For this review, take the finished solid that the model builds, in its own axes (mm). Face numbers are marked on the shaded views. A direction names the side the tool comes from. Round coordinates to 2 decimals unless told otherwise and drop trailing zeros. Write each loop counter-clockwise with the first axis right and the second up, starting at its lowest first coordinate (ties: lowest second). Pieces come first, ordered by that corner, then holes. Notation, with made-up numbers: (-22, 18.5) -> (0, 18.5) arc R9 cw to (0, 27.5) -> close; hole circle Ø6 at (-15, -9.5). An arc over 180 degrees is marked (long way). Answer in a Markdown table with one row per item. Add a question column.
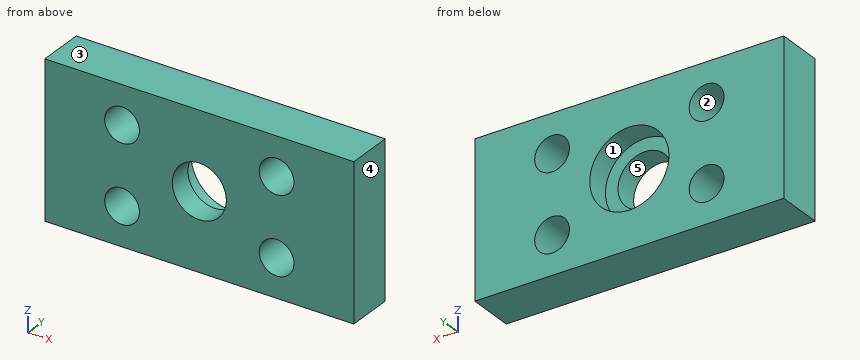
```python
from build123d import *

# Parameters (mm, degrees)
SKETCH_2_W          = 120
SKETCH_2_H          = 20
SKETCH_2_R          = 2.25
EXTRUDE_1_DEPTH     = 6
SKETCH_3_W          = 80
SKETCH_3_H          = 20
CUT_EXTRUDE_1_DEPTH = 62.12282716
SKETCH_4_R          = 5.125
CUT_EXTRUDE_2_DEPTH = 3
SKETCH_5_R          = 3.5
CUT_EXTRUDE_3_DEPTH = 61.901559914


with BuildPart() as part:
    # Эскиз2 → Бобышка-Вытянуть1 (new body)
    with BuildSketch(Plane(origin=(0, 0, 0), x_dir=(1, 0, 0), z_dir=(0, 1, 0))):
        Rectangle(SKETCH_2_W, SKETCH_2_H)
        with Locations(Location((-50, 5, 0), (0, 0, 270))):
            Circle(SKETCH_2_R, mode=Mode.SUBTRACT)
        with Locations(Location((-30, 5, 0), (0, 0, 270))):
            Circle(SKETCH_2_R, mode=Mode.SUBTRACT)
        with Locations(Location((-10, 5, 0), (0, 0, 270))):
            Circle(SKETCH_2_R, mode=Mode.SUBTRACT)
        with Locations(Location((30, 5, 0), (0, 0, 270))):
            Circle(SKETCH_2_R, mode=Mode.SUBTRACT)
        with Locations(Location((-30, -5, 0), (0, 0, 270))):
            Circle(SKETCH_2_R, mode=Mode.SUBTRACT)
        with Locations(Location((10, -5, 0), (0, 0, 270))):
            Circle(SKETCH_2_R, mode=Mode.SUBTRACT)
        with Locations(Location((50, -5, 0), (0, 0, 270))):
            Circle(SKETCH_2_R, mode=Mode.SUBTRACT)
        with Locations(Location((-50, -5, 0), (0, 0, 270))):
            Circle(SKETCH_2_R, mode=Mode.SUBTRACT)
    extrude(amount=EXTRUDE_1_DEPTH)

    # Эскиз3 → Вырез-Вытянуть1 (cut, through all)
    with BuildSketch(Plane(origin=(0, 6, 0), x_dir=(1, 0, 0), z_dir=(0, 1, 0))):
        with Locations((20, 0)):
            Rectangle(SKETCH_3_W, SKETCH_3_H)
    extrude(amount=-CUT_EXTRUDE_1_DEPTH, mode=Mode.SUBTRACT)

    # Эскиз4 → Вырез-Вытянуть2 (cut)
    with BuildSketch(Plane(origin=(0, 6, 0), x_dir=(1, 0, 0), z_dir=(0, 1, 0))):
        with Locations(Location((-40, 0, 0), (0, 0, 270))):
            Circle(SKETCH_4_R)
    extrude(amount=-CUT_EXTRUDE_2_DEPTH, mode=Mode.SUBTRACT)

    # Эскиз5 → Вырез-Вытянуть3 (cut, through all)
    with BuildSketch(Plane(origin=(0, 3, 0), x_dir=(1, 0, 0), z_dir=(0, 1, 0))):
        with Locations(Location((-40, 0, 0), (0, 0, 270))):
            Circle(SKETCH_5_R)
    extrude(amount=-CUT_EXTRUDE_3_DEPTH, mode=Mode.SUBTRACT)


solid = part.part
```
1. We need section A-A (x = -40). Write out the cut boundary in (y, z) (3 decimals), plus the area to 4 significant figures.
2. We need section D-D (x = -50). Write out the cut boundary in (y, z), plus the area to 3 significant figures.
3. Clearance check with flat-ended pins moving along their axes: pin 1 Ø5.5 at (x, z) = (-40, 0) entering from +Y; pin 2 Ø9 at (x, z) = (-40, 0) entering from +Y. State where each tip first meets the part, or that it passes through.
4. For L1, parallel to X at y = 1.8, z = -5; L2, parallel to X at y = 2.1, z = -6.5; L3, parallel to X at y = 1.8, z = 0, list the stretches that pass through material, from the lowest coordinate up. Write a range as [from, to].
5. The part is to be moulded in two halves that separate along X. For the marked faces 3, 4 and 5, say which applies: pulls with the +X half, pulls with the -X half, needs draft (parallel to the pull), parting line crosses it, or undercut.
6. We need section B-B (y = 1.65). Write out the cut boundary in (x, z), plus the area to 3 significant figures.
7. We need section C-C (z = 0). Write out the cut boundary in (x, y) (3 decimals).
8. Tool access review of the marked faces 1 and 2: name each direction out of +Z, -Z, +X, -X, +Y, -Y from which nothing blocks a thin tool from reaching the whole face with its end or side.
Response:
| question | item | result |
|---|---|---|
| 1 | outline | (0, -10) -> (6, -10) -> (6, -5.125) -> (3, -5.125) -> (3, -3.5) -> (0, -3.5) -> close; (0, 3.5) -> (3, 3.5) -> (3, 5.125) -> (6, 5.125) -> (6, 10) -> (0, 10) -> close |
| 1 | area | 68.25 mm2 |
| 2 | outline | (0, -10) -> (6, -10) -> (6, -7.25) -> (0, -7.25) -> close; (0, -2.75) -> (6, -2.75) -> (6, 2.75) -> (0, 2.75) -> close; (0, 7.25) -> (6, 7.25) -> (6, 10) -> (0, 10) -> close |
| 2 | area | 66.0 mm2 |
| 3 | pin 1 | through |
| 3 | pin 2 | y = 3 |
| 4 | L1 | [-60, -52.25], [-47.75, -32.25], [-27.75, -20] |
| 4 | L2 | [-60, -51.68], [-48.32, -31.68], [-28.32, -20] |
| 4 | L3 | [-60, -43.5], [-36.5, -20] |
| 5 | face 3 | needs draft |
| 5 | face 4 | pulls with the +X half |
| 5 | face 5 | undercut |
| 6 | outline | (-60, -10) -> (-20, -10) -> (-20, 10) -> (-60, 10) -> close; hole circle Ø4.5 at (-50, -5); hole circle Ø4.5 at (-50, 5); hole circle Ø7 at (-40, 0); hole circle Ø4.5 at (-30, -5); hole circle Ø4.5 at (-30, 5) |
| 6 | area | 698 mm2 |
| 7 | outline | (-60, 0) -> (-43.5, 0) -> (-43.5, 3) -> (-45.125, 3) -> (-45.125, 6) -> (-60, 6) -> close; (-36.5, 0) -> (-20, 0) -> (-20, 6) -> (-34.875, 6) -> (-34.875, 3) -> (-36.5, 3) -> close |
| 8 | face 1 | +Y |
| 8 | face 2 | +Y, -Y |
